Model file for the job. Use its own axes, mm. Coordinates: 2 decimals unless noted, no trailing zeros. Order: outer loops, then holes, each group sorted by start corner. A loop starts at its lowest first (then second) coordinate and runs counter-clockwise, first axis right, second up.
from build123d import *

# Parameters (mm, degrees)
SKETCH_1_W          = 60
SKETCH_1_H          = 60.44
SKETCH_1_R          = 2.75
EXTRUDE_1_DEPTH     = 4
SKETCH_3_R          = 20
CUT_EXTRUDE_1_DEPTH = 5
SKETCH_6_W          = 60
SKETCH_6_H          = 4
EXTRUDE_2_DEPTH     = 10


with BuildPart() as part:
    # 草圖1 → 填料-伸長1 (new body)
    with BuildSketch(Plane.XY):
        with Locations((30, -30.22)):
            Rectangle(SKETCH_1_W, SKETCH_1_H)
        with Locations((5.25, -5.25)):
            Circle(SKETCH_1_R, mode=Mode.SUBTRACT)
        with Locations((54.75, -5.25)):
            Circle(SKETCH_1_R, mode=Mode.SUBTRACT)
        with Locations((5.25, -54.75)):
            Circle(SKETCH_1_R, mode=Mode.SUBTRACT)
        with Locations((54.75, -54.75)):
            Circle(SKETCH_1_R, mode=Mode.SUBTRACT)
    extrude(amount=EXTRUDE_1_DEPTH)

    # 草圖3 → 除料-伸長1 (cut, through all)
    with BuildSketch(Plane.XY.offset(4)):
        with Locations((30, -34.716194978)):
            Circle(SKETCH_3_R)
    extrude(amount=-CUT_EXTRUDE_1_DEPTH, mode=Mode.SUBTRACT)

    # 草圖6 → 填料-伸長2 (add)
    with BuildSketch(Plane(origin=(0, 0, 0), x_dir=(1, 0, 0), z_dir=(0, 1, 0))):
        with Locations((30, -2)):
            Rectangle(SKETCH_6_W, SKETCH_6_H)
    extrude(amount=EXTRUDE_2_DEPTH)


solid = part.part
Q1. Probe line 1 (Y direction, x = 5.25, z = 0.8); line 2 (X direction, y = -55, z = 1.3); line 3 (X direction, y = -34.5, z = 0.25). List the from-to ranges inside material, lowest first.
Established:
line 1: y = -60.44 to -57.5, -52 to -8, -2.5 to 10
line 2: x = 0 to 2.51, 7.99 to 52.01, 57.49 to 60
line 3: x = 0 to 10, 50 to 60
Q2. Cut at A-A, the plane x = 30. List the corners of the cut face in (y, z), plus the area to 3 significant figures.
Established:
outline: (-60.44, 0) - (-54.72, 0) - (-54.72, 4) - (-60.44, 4) - close; (-14.72, 0) - (10, 0) - (10, 4) - (-14.72, 4) - close
area: 122 mm2
Q3. Cut at D-D, the plane z = 2.7. List the corners of the cut face in (x, y), plus the area to 3 significant figures.
Established:
outline: (0, -60.44) - (60, -60.44) - (60, 10) - (0, 10) - close; hole circle Ø5.5 at (5.25, -54.75); hole circle Ø5.5 at (5.25, -5.25); hole circle Ø40 at (30, -34.72); hole circle Ø5.5 at (54.75, -54.75); hole circle Ø5.5 at (54.75, -5.25)
area: 2,870 mm2
Q4. Mould opens along Y. For faces 1 (the face through (30, -60.44, 2)), 2 (the face through (60, -26, 2)), 3 (the face through (4.892, -52.023, 1.972)) say: pulls with the +Y half, pulls with the -Y half, needs draft (parallel to the pull), parting line crosses it, or undercut.
Established:
face 1: pulls with the -Y half
face 2: needs draft
face 3: undercut
Q5. Cut at B-B, the plane y = -37.5. List the corners of the cut face in (x, z).
Established:
outline: (0, 0) - (10.19, 0) - (10.19, 4) - (0, 4) - close; (49.81, 0) - (60, 0) - (60, 4) - (49.81, 4) - close
Q6. Cut at C-C, the plane x = 5.25. List the corners of the cut face in (y, z).
Established:
outline: (-60.44, 0) - (-57.5, 0) - (-57.5, 4) - (-60.44, 4) - close; (-52, 0) - (-8, 0) - (-8, 4) - (-52, 4) - close; (-2.5, 0) - (10, 0) - (10, 4) - (-2.5, 4) - close
